Could you check a few things on this model? Use its own coordinates, in mm. A direction names the side the tool comes from. Coordinates: 2 decimals unless noted, no trailing zeros. Loops run counter-clockwise (first coordinate to the right, second up) from the corner with the lowest first, then second, coordinate; pieces in that order, holes last. Notation, with made-up numbers: (6.5, -4.75) -> (26.5, -4.75) arc R4 cw to (26.5, 1.25) -> close; hole circle Ø7 at (42, 38.5). An arc over 180 degrees is marked (long way). One line per question, with ' | ' between items.
from build123d import *

# Parameters (mm, degrees)
SKETCH1_R           = 5.1
BOSS_EXTRUDE1_DEPTH = 10
CUT_EXTRUDE1_REACH  = 111.4


with BuildPart() as part:
    # Sketch1 → Boss-Extrude1 (new body)
    with BuildSketch(Plane.XY):
        Polygon((-3.661981052, -82.908158574), (70.673174696, -33.455495228), (26.915653686, 32.318962998), (-47.419502062, -17.133700347), align=None)
        Circle(SKETCH1_R, mode=Mode.SUBTRACT)
        with Locations((34.929606693, 2.218687963)):
            Circle(SKETCH1_R, mode=Mode.SUBTRACT)
        with Locations((54.315850178, -26.921894796)):
            Circle(SKETCH1_R, mode=Mode.SUBTRACT)
        with Locations((23.253672634, -50.589195576)):
            Circle(SKETCH1_R, mode=Mode.SUBTRACT)
        with Locations((-11.675934059, -52.807883539)):
            Circle(SKETCH1_R, mode=Mode.SUBTRACT)
        with Locations((-31.062177544, -23.66730078)):
            Circle(SKETCH1_R, mode=Mode.SUBTRACT)
    extrude(amount=-BOSS_EXTRUDE1_DEPTH)

    # Sketch2 → Cut-Extrude1 (cut, up to next)
    with BuildSketch(Plane.XY, mode=Mode.PRIVATE) as cut_extrude1_sk1:
        Polygon((4.322740293, -20.01253557), (19.311853758, -20.583917696), (18.930932341, -30.576660006), (3.941818876, -30.00527788), align=None)
    cut_extrude1_tool1 = extrude(cut_extrude1_sk1.sketch, amount=-CUT_EXTRUDE1_REACH, mode=Mode.PRIVATE) & part.part
    add(cut_extrude1_tool1.solids().sort_by_distance((11.626836, -25.294598, 0))[0], mode=Mode.SUBTRACT)


solid = part.part
1) We'd pull the mould along Y, two halves only. Please class faces 1 (the face through (-25.847, -49.561, -4.93)), 2 (the face through (4.13, -25.08, -4.93)), 3 (the face through (49.1, -1.03, -4.93)): pulls with the +Y half, pulls with the -Y half, needs draft (parallel to the pull), parting line crosses it, or undercut.
Data:
face 1: pulls with the -Y half | face 2: undercut | face 3: pulls with the +Y half
2) If we section it at B-B on y = 0: Please give me the cut outline in (x, z).
Data:
outline: (-21.66, -10) -> (-5.1, -10) -> (-5.1, 0) -> (-21.66, 0) -> close; (5.1, -10) -> (30.34, -10) -> (30.34, 0) -> (5.1, 0) -> close; (39.52, -10) -> (48.42, -10) -> (48.42, 0) -> (39.52, 0) -> close
3) I need wall thicknesses on line 1 along X through (y, z) = (0.5, -1.5); line 2 along X through (y, z) = (-26.5, -8.5); line 3 along X through (y, z) = (-21, -9.5). Which ranges of each line are inside material? Lowest first, please. Write a range as from..to.
Data:
line 1: -20.91..-5.08, 5.08..30.13, 39.73..48.08 | line 2: -41.19..-35.3, -26.82..4.08, 19.09..49.23, 59.4..66.05 | line 3: -44.85..-35.41, -26.72..4.29, 19.3..62.39
4) I'm going to push flat-ended pins straight in: pin 1 Ø1 at (x, z) = (58.5, -8.5) entering from -Y; pin 2 Ø2 at (x, z) = (41, -6.5) entering from -Y; pin 3 Ø3 at (y, z) = (0.5, -2.5) entering from +X. Where does each tip first touch, or does it pass through?
Data:
pin 1: y = -41.89 | pin 2: y = -53.86 | pin 3: x = 49.08
5) On a 3-axis mill with a long thin cutter (end or side, diameter ignored), from which of +Z, -Z, +X, -X, +Y, -Y can I reach the whole of each face in a straight line? I mean faces 4 (the face through (11.541, -30.295, -4.93)), 5 (the face through (32.985, -58.528, -4.93)). Say none if no direction works.
Data:
face 4: +Z, -Z | face 5: +Z, -Z, +X, -Y
6) If we section it at C-C on z = -7.5: Please give me the cut outline in (x, y), and give its area (3 significant figures).
Data:
outline: (-47.42, -17.13) -> (-3.66, -82.91) -> (70.67, -33.46) -> (26.92, 32.32) -> close; hole circle Ø10.2 at (-31.06, -23.67); hole circle Ø10.2 at (-11.68, -52.81); hole circle Ø10.2 at (0, 0); hole (3.94, -30.01) -> (18.93, -30.58) -> (19.31, -20.58) -> (4.32, -20.01) -> close; hole circle Ø10.2 at (23.25, -50.59); hole circle Ø10.2 at (34.93, 2.22); hole circle Ø10.2 at (54.32, -26.92) | area: 6,410 mm²
7) If we section it at D-D on x = 56: Please give me the cut outline in (y, z).
Data:
outline: (-43.22, -10) -> (-31.74, -10) -> (-31.74, 0) -> (-43.22, 0) -> close; (-22.11, -10) -> (-11.4, -10) -> (-11.4, 0) -> (-22.11, 0) -> close
8) If we section it at A-A on x = 0: Please give me the cut outline in (y, z), and give its area (3 significant figures).
Data:
outline: (-80.47, -10) -> (-5.1, -10) -> (-5.1, 0) -> (-80.47, 0) -> close; (5.1, -10) -> (14.41, -10) -> (14.41, 0) -> (5.1, 0) -> close | area: 847 mm²
